Drawing for the job (mm, zero at the part's lowest x, y, z). A direction names the side the tool comes from. Give positions to 0.01 mm unless a question says otherwise; leave off trailing zeros. Order: outer loops, then holes, each group sorted by start corner. A loop starts at its lowest first (then second) coordinate and runs counter-clockwise, first axis right, second up. Notation, with made-up numbers: (89, 74) - (129, 74) arc R19 ccw to (129, 96) - close; hole circle Ø8 at (52.5, 88). An arc over 180 degrees is marked (long way). One line per item, written item: value.
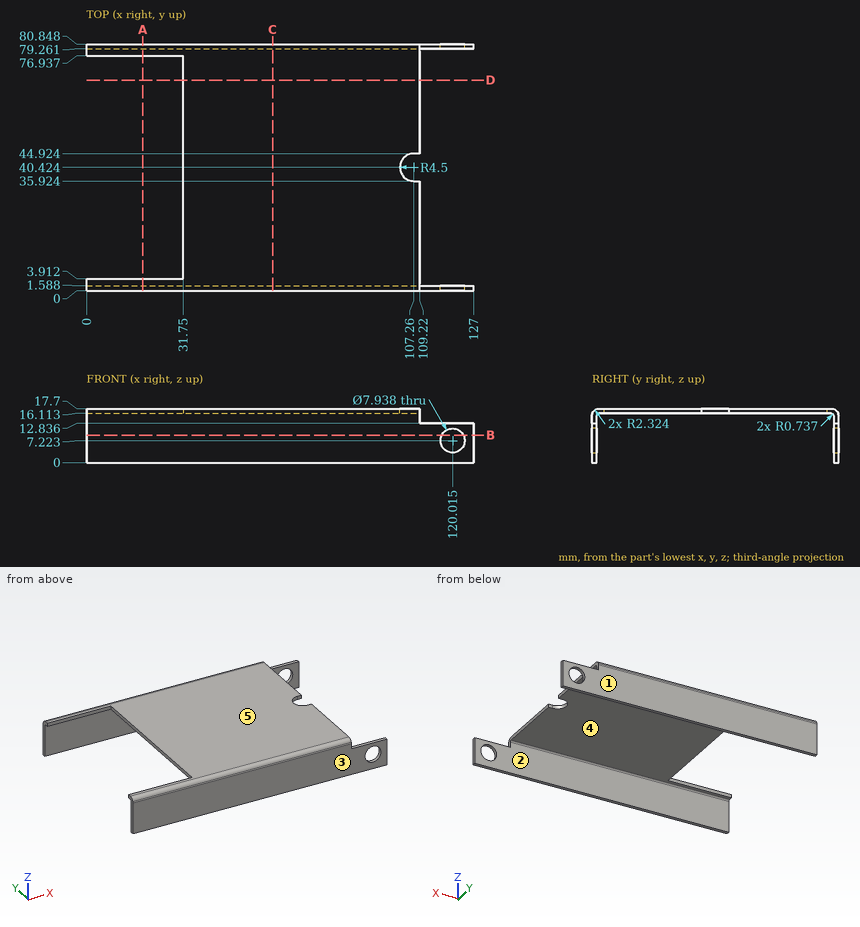
1) Which spindle directions (+Z, -Z, +X, -X, +Y, -Y) get a long thin tool onto all of the face, cutting with end or side? Do the marked faces 4 and 5. Say none if no direction does.
Outcome:
face 4: -Z, +X, -X
face 5: +Z, +X, -X, +Y, -Y
2) Pin check, flat tips, straight feed: pin 1 (0.8 mm diameter, centred on x = 122.5, y = 1, fed in from +Z); pin 2 (1.7 mm diameter, centred on x = 9.5, z = 17, fed in from -Y); pin 3 (0.8 mm diameter, centred on x = 13, z = 17, fed in from +Y). Stop position of each tip, or through.
Outcome:
pin 1: stops at z = 12.84
pin 2: stops at y = 0.13
pin 3: stops at y = 80.5
3) Drill centre lines: line 1 along Y through (x, z) = (29, 6.25); line 2 along Z through (x, y) = (56, 75). Where is each one in solid material? Low to high. Write a range as from..to.
Outcome:
line 1: y = 0..1.59, 79.26..80.85
line 2: z = 16.11..17.7
4) Mould opens along Y. For the marked faces 1, 2 and 3 say: released by +Y, released by -Y, zero draft, split by the parting line, or undercut.
Outcome:
face 1: released by +Y
face 2: undercut
face 3: released by -Y
5) Cut at D-D, the plane y = 69. Give the cut face in (x, z).
Outcome:
outline: (31.75, 16.11) - (109.22, 16.11) - (109.22, 17.7) - (31.75, 17.7) - close
6) Cut at A-A, the plane x = 18.5. Give the cut face in (y, z) (1 decimal).
Outcome:
outline: (0, 0) - (1.6, 0) - (1.6, 15.4) arc R0.7 cw to (2.3, 16.1) - (3.9, 16.1) - (3.9, 17.7) - (2.3, 17.7) arc R2.3 ccw to (0, 15.4) - close; (76.9, 16.1) - (78.5, 16.1) arc R0.7 cw to (79.3, 15.4) - (79.3, 0) - (80.8, 0) - (80.8, 15.4) arc R2.3 ccw to (78.5, 17.7) - (76.9, 17.7) - close
7) Cut at C-C, the plane x = 61. Give the cut face in (y, z) (1 decimal).
Outcome:
outline: (0, 0) - (1.6, 0) - (1.6, 15.4) arc R0.7 cw to (2.3, 16.1) - (78.5, 16.1) arc R0.7 cw to (79.3, 15.4) - (79.3, 0) - (80.8, 0) - (80.8, 15.4) arc R2.3 ccw to (78.5, 17.7) - (2.3, 17.7) arc R2.3 ccw to (0, 15.4) - close
8) Cut at B-B, the plane z = 9. Give the cut face in (x, y).
Outcome:
outline: (0, 0) - (116.47, 0) - (116.47, 1.59) - (0, 1.59) - close; (0, 79.26) - (116.47, 79.26) - (116.47, 80.85) - (0, 80.85) - close; (123.56, 0) - (127, 0) - (127, 1.59) - (123.56, 1.59) - close; (123.56, 79.26) - (127, 79.26) - (127, 80.85) - (123.56, 80.85) - close
